Check sheet for the modelled part. Datum: model origin and axes. Units: mm. Face numbers are marked on the shaded views. Round coordinates to 2 decimals unless told otherwise and drop trailing zeros. Write each loop counter-clockwise with the first axis right and the second up, starting at its lowest first coordinate (ties: lowest second). Pieces come first, ordered by that corner, then holes. Notation, with made-up numbers: (72.5, 52.5) -> (107.5, 52.5) arc R6 cw to (107.5, 60.5) -> close; hole circle Ø10 at (-10.5, 9.5). An arc over 180 degrees is marked (long way). Answer as a JSON object with one key per item and string values. Group by question number.
```python
from build123d import *

# Parameters (mm, degrees)
SKETCH1_R           = 3.175
SKETCH1_R_2         = 1.27
BOSS_EXTRUDE2_DEPTH = 2.54


with BuildPart() as part:
    # Sketch1 → Boss-Extrude2 (new body)
    # profile 1 of 3: a face of its own
    with BuildSketch(Plane.XY):
        Circle(SKETCH1_R)
        Circle(SKETCH1_R_2, mode=Mode.SUBTRACT)
    # profile 2 of 3: a face of its own
    with BuildSketch(Plane.XY):
        with Locations((25.9207, 0)):
            Circle(SKETCH1_R)
        with Locations((25.9207, 0)):
            Circle(SKETCH1_R_2, mode=Mode.SUBTRACT)
    # profile 3 of 3: a face of its own
    with BuildSketch(Plane.XY):
        with BuildLine():
            Line((25.9207, 3.175), (0, 3.175))
            ThreePointArc((0, 3.175), (2.24506403, 2.24506403), (3.175, 0))
            ThreePointArc((3.175, 0), (2.24506403, -2.24506403), (0, -3.175))
            Line((0, -3.175), (25.9207, -3.175))
            ThreePointArc((25.9207, -3.175), (22.7457, 0), (25.9207, 3.175))
        make_face()
    extrude(amount=BOSS_EXTRUDE2_DEPTH)


solid = part.part
```
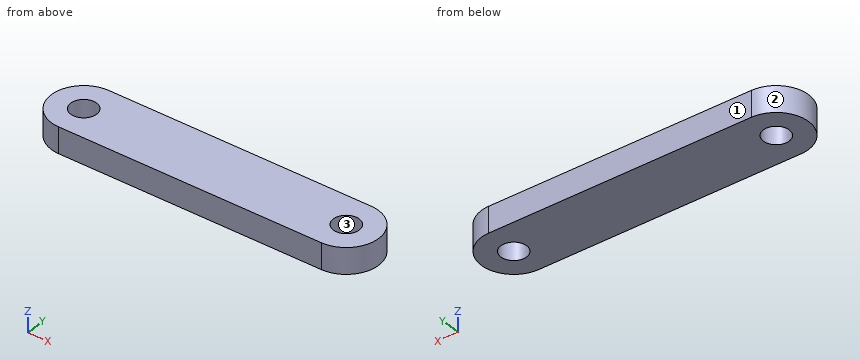
(1) Section check C-C on y = -2.5. Record the cut outline in (x, z), then the cut area to 3 significant figures.
(2) Section check A-A on y = 0. Record the cut outline in (x, z) (3 decimals), then the cut area to 3 significant figures.
(3) Section check B-B on z = 0.65. Record the cut outline in (x, y) (3 decimals), then the cut area to 3 significant figures.
(4) Release check for a two-part mould opening along X. For the marked faces 1, 2 and 3 record: pulls with the +X half, pulls with the -X half, needs draft (parallel to the pull), parting line crosses it, or undercut.
(5) Scan lines: line 1 along X through (y, z) = (0.5, 0.5); line 2 along X through (y, z) = (-0.25, 1.25); line 3 along X through (y, z) = (-1.5, 1.45). Record each from-to range of solid material in increasing order.
(6) Go/stop test with flat-tipped pins: pin 1 Ø1.5 at (y, z) = (2.5, 2) entering from +X; pin 2 Ø1.5 at (y, z) = (2, 0.5) entering from +X. Record where each tip stops, or that it passes through.
Data:
{
 "1": {"outline": "(-1.96, 0) -> (27.88, 0) -> (27.88, 2.54) -> (-1.96, 2.54) -> close", "area": "75.8 mm²"},
 "2": {"outline": "(-3.175, 0) -> (-1.27, 0) -> (-1.27, 2.54) -> (-3.175, 2.54) -> close; (1.27, 0) -> (24.651, 0) -> (24.651, 2.54) -> (1.27, 2.54) -> close; (27.191, 0) -> (29.096, 0) -> (29.096, 2.54) -> (27.191, 2.54) -> close", "area": "69.1 mm²"},
 "3": {"outline": "(0, -3.175) -> (25.921, -3.175) arc R3.175 ccw to (25.921, 3.175) -> (0, 3.175) arc R3.175 ccw to start; hole circle Ø2.54 at (0, 0); hole circle Ø2.54 at (25.921, 0)", "area": "186 mm²"},
 "4": {"face 1": "needs draft", "face 2": "pulls with the -X half", "face 3": "undercut"},
 "5": {"line 1": "x = -3.14 to -1.17, 1.17 to 24.75, 27.09 to 29.06", "line 2": "x = -3.17 to -1.25, 1.25 to 24.68, 27.17 to 29.09", "line 3": "x = -2.8 to 28.72"},
 "6": {"pin 1": "stops at x = 28.57", "pin 2": "stops at x = 28.84"}
}
